Part model, mm, in its own coordinate system. A direction names the side the tool comes from. Coordinates: 2 decimals unless noted, no trailing zeros. One line per question, with ' | ' between items. Start each with the question number.
1) Probe L1, parallel to Z at x = -5, y = -12.5; L2, parallel to Z at x = -6.5, y = -12.5; L3, parallel to Z at x = -5, y = 18. List the from-to ranges inside material, lowest first. Write a range as from..to.
2) Two-plate mould, pull along Z, no slides. Class faces 3 (the face through (8.484, -12.629, -2.672)), 4 (the face through (-8, -19, -1.984)), 5 (the face through (0, -25, 0)), 6 (the face through (6.831, -19, 0)): released by +Z, released by -Z, zero draft, split by the parting line, or undercut.
3) Drop flat-ended pins along their axis: pin 1 (2 mm diameter, centred on x = 8, y = -17.5, fed in from +Z); pin 2 (4 mm diameter, centred on y = 9, z = -3.5, fed in from +X); pin 3 (0.6 mm diameter, centred on x = -8, y = -17.5, fed in from -Z); pin 4 (2.5 mm diameter, centred on y = -12.5, z = 0, fed in from +X). Give the stop position or say it passes through.
4) 3-axis set-ups, long thin cutter, end or side, ignore diameter. For faces 1 (the face through (8, -19, -1.984)), 2 (the face through (-8, -19, 1.984)): which of +Z, -Z, +X, -X, +Y, -Y reach the whole face in a straight line?
from build123d import *

# Parameters (mm, degrees)
SKETCH1_R               = 8.895
BOSS_EXTRUDE1_DEPTH     = 25
CUT_EXTRUDE1_DEPTH      = 12.5
SKETCH3_R               = 1.984375
CUT_EXTRUDE2_DEPTH      = 9.895
CUT_EXTRUDE2_DEPTH_BACK = 9.895
CHAMFER1_SIZE           = 0.6


with BuildPart() as part:
    # Sketch1 → Boss-Extrude1 (new body)
    with BuildSketch(Plane(origin=(0, 0, 0), x_dir=(1, 0, 0), z_dir=(0, 1, 0))):
        Circle(SKETCH1_R)
    extrude(amount=-BOSS_EXTRUDE1_DEPTH)

    # Sketch2 → Cut-Extrude1 (cut)
    with BuildSketch(Plane.XZ.offset(25)):
        with BuildLine():
            Line((-6.83125, 1.984375), (-6.83125, -1.984375))
            Line((-6.83125, -1.984375), (-8.670829306, -1.984375))
            ThreePointArc((-8.670829306, -1.984375), (-8.895, 0), (-8.670829306, 1.984375))
            Line((-8.670829306, 1.984375), (-6.83125, 1.984375))
        make_face()
    cut_extrude1 = extrude(amount=-CUT_EXTRUDE1_DEPTH, mode=Mode.SUBTRACT)

    # Mirror1: Cut-Extrude1 across plane
    add(cut_extrude1.mirror(Plane(origin=(0, 0, 0), x_dir=(0, 0, 1), z_dir=(1, 0, 0))), mode=Mode.SUBTRACT)

    # Sketch3 → Cut-Extrude2 (cut, two sides)
    with BuildSketch(Plane(origin=(0, 0, 0), x_dir=(0, 0, -1), z_dir=(1, 0, 0))) as cut_extrude2_sk:
        with Locations((0, -12.5)):
            Circle(SKETCH3_R)
    extrude(amount=CUT_EXTRUDE2_DEPTH, mode=Mode.SUBTRACT)
    extrude(cut_extrude2_sk.sketch, amount=-CUT_EXTRUDE2_DEPTH_BACK, mode=Mode.SUBTRACT)

    # Sketch4 → Revolve1 (revolve)
    with BuildSketch(Plane.XY):
        with BuildLine():
            Line((0, 0), (0, 76.2))
            add(Edge.make_bspline(
                [(0, 76.2), (0.010785041, 76.199224813), (0.031898851, 76.195655683), (0.072292948, 76.180192568), (0.120867926, 76.149408415), (0.16893656, 76.109505667), (0.219506214, 76.05859599), (0.270891595, 75.999075831), (0.33405813, 75.915307947), (0.416902674, 75.788683792), (0.530129314, 75.587496608), (0.690806004, 75.250371079), (0.925151077, 74.660400515), (1.28066013, 73.56410381), (1.819345698, 71.484532143), (2.494562294, 68.169675275), (3.229107388, 63.761120823), (3.974148921, 58.507567912), (4.671648215, 52.966650055), (5.309955775, 47.384032694), (5.89808978, 41.850390189), (6.456372381, 36.225635174), (6.974392848, 30.74087905), (7.485193122, 25.019380562), (7.946052453, 19.68165029), (8.436147301, 13.706913443), (8.831540425, 8.78213491), (9.214950637, 3.783393938), (9.405019243, 1.269742765), (9.500000001, 0)],
                knots=[0, 0, 0, 0, 0, 0.000506263, 0.001012527, 0.002025053, 0.002702132, 0.00345017, 0.004398317, 0.005734537, 0.007654734, 0.010586496, 0.015298636, 0.023344234, 0.03763286, 0.06493253, 0.116773094, 0.182858951, 0.248944817, 0.315030683, 0.381116549, 0.447202415, 0.513288281, 0.579374148, 0.645460014, 0.71154588, 0.777631747, 0.843717613, 0.909803479, 0.909803479, 0.909803479, 0.909803479, 0.909803479], degree=4))
            Line((9.500000001, 0), (0, 0))
        make_face()
    revolve(axis=Axis((0, 0, 0), (0, 1, 0)))

    # Chamfer1
    chamfer1_edges = [part.edges().sort_by_distance(p)[0] for p in [
        (-8.895, 0, 0),
    ]]
    chamfer(chamfer1_edges, length=CHAMFER1_SIZE)


solid = part.part
Reported:
1) L1: z = -7.36..-1.98, 1.98..7.36 | L2: z = -6.07..-1.98, 1.98..6.07 | L3: z = -6.35..6.35
2) face 3: split by the parting line | face 4: undercut | face 5: zero draft | face 6: undercut
3) pin 1: stops at z = 5.49 | pin 2: stops at x = 8.71 | pin 3: stops at z = -4.45 | pin 4: passes through
4) face 1: +X, -Y | face 2: -X, -Y
